from build123d import *

# Parameters (mm, degrees)
F1_DEPTH = 12.7


with BuildPart() as f1:
    # F0 (on Top) → F1 (new body)
    with BuildSketch(Plane.XY):
        with BuildLine():
            Line((-571.475674, 0), (0, 0))
            Line((0, 0), (0, 12.7))
            Line((0, 12.7), (-533.4, 25.4))
            Line((-533.4, 25.4), (-546.1, 25.4))
            ThreePointArc((-546.1, 25.4), (-579.054577, 34.270767), (-609.6, 19.05))
            Line((-609.6, 19.05), (-577.85, 19.05))
            ThreePointArc((-577.85, 19.05), (-573.111527, 10.044084), (-571.475674, 0))
        make_face()
        with BuildLine():
            Line((0, -12.7), (0, 0))
            Line((0, 0), (-571.475674, 0))
            ThreePointArc((-571.475674, 0), (-573.111527, -10.044084), (-577.85, -19.05))
            Line((-577.85, -19.05), (-609.6, -19.05))
            ThreePointArc((-609.6, -19.05), (-579.054577, -34.270767), (-546.1, -25.4))
            Line((-546.1, -25.4), (-533.4, -25.4))
            Line((-533.4, -25.4), (0, -12.7))
        make_face()
    extrude(amount=F1_DEPTH)


solid = f1.part
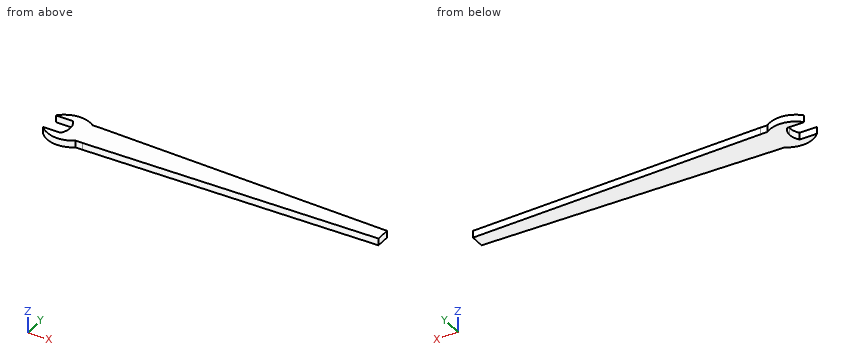
Verification items for the finished model (mm, model axes). Coordinates: 2 decimals unless noted, no trailing zeros. Order: outer loops, then holes, each group sorted by start corner. A loop starts at its lowest first (then second) coordinate and runs counter-clockwise, first axis right, second up. Notation, with made-up numbers: M 48,7.5 L 91,7.5 A31 cw 91,34.5 Z; hole C -30,44.5 d10. An arc over 180 degrees is marked long. One line per item, written item: value. Start each with the question number.
Item 1: Thickness scan on probe 1 along X at (y, z) = (2.5, 12.25); probe 2 along X at (y, z) = (6.5, 8.75); probe 3 along Y at (x, z) = (-215.5, 8.5). Record the ranges inside material, lowest first.
Item 2: Sectioned sample at A-A on z = 7.5. Record the cut outline in (x, y).
Item 3: Depth check by flat-ended pin: P1, Ø1.5, axis at y = 15.5, z = 11, coming from the -X side; P2, Ø5, axis at x = -142.5, z = 7.5, coming from the +Y side; P3, Ø1, axis at y = -6.5, z = 5, coming from the -X side. Enter the tip coordinate at first touch or a pass-through.
Item 4: Sectioned sample at C-C on x = -254. Record the cut outline in (y, z).
Item 5: Sectioned sample at B-B on x = -75.5. Record the cut outline in (y, z), then the cut area to 3 significant figures.
Calculated:
1. probe 1: -571.57 to 0
1. probe 2: -572.15 to 0
1. probe 3: -17.83 to 17.83
2. outline: M -609.6,-19.05 A48.1 ccw -546.1,-25.4 L -533.4,-25.4 L 0,-12.7 L 0,12.7 L -533.4,25.4 L -546.1,25.4 A48.1 ccw -609.6,19.05 L -577.85,19.05 A31.65 cw -571.48,0 A31.65 cw -577.85,-19.05 Z
3. P1: x = -575.97
3. P2: y = 16.15
3. P3: x = -572.26
4. outline: M -18.75,0 L 18.75,0 L 18.75,12.7 L -18.75,12.7 Z
5. outline: M -14.5,0 L 14.5,0 L 14.5,12.7 L -14.5,12.7 Z
5. area: 368 mm^2
